For this review, take the finished solid that the model builds, in its own axes (mm). A direction names the side the tool comes from. Give positions to 0.01 mm unless a question says otherwise; leave off trailing zeros. Loops run counter-clockwise (first coordinate to the right, second up) from the corner with the lowest first, then second, coordinate; pieces in that order, holes last. Notation, with made-up numbers: (84.5, 72.5) - (141.5, 72.5) arc R24 ccw to (141.5, 98.5) - close; hole circle Ø1 at (26.25, -16.75). An arc over 180 degrees is marked (long way). Put each result on its own line as item: value.
from build123d import *

# Parameters (mm, degrees)
ESQUISSE1_R             = 1.75
ESQUISSE1_R_2           = 3.5
BOSS_EXTRU_1_DEPTH      = 5
ENL_V_MAT_EXTRU_2_REACH = 41.592
BOSS_EXTRU_2_DEPTH      = 30
ESQUISSE5_W             = 30
ESQUISSE5_H             = 5
BOSS_EXTRU_3_DEPTH      = 20
BOSS_EXTRU_4_DEPTH      = 2
BOSS_EXTRU_5_DEPTH      = 2
ENL_V_MAT_EXTRU_3_REACH = 42.516
ESQUISSE12_R            = 1.75
BOSS_EXTRU_6_DEPTH      = 4
BOSS_EXTRU_6_DEPTH_BACK = 4


with BuildPart() as part:
    # Esquisse1 → Boss.-Extru.1 (new body)
    with BuildSketch(Plane.XY):
        with BuildLine():
            Line((-15.959557324, 10.348837209), (-15.959557324, -9.651162791))
            Line((-15.959557324, -9.651162791), (14.040442676, -9.651162791))
            Line((14.040442676, -9.651162791), (14.040442676, 10.348837209))
            ThreePointArc((14.040442676, 10.348837209), (-0.959557324, 25.348837209), (-15.959557324, 10.348837209))
        make_face()
        with Locations((-8.959557324, 10.348837209)):
            Circle(ESQUISSE1_R, mode=Mode.SUBTRACT)
        with Locations((7.040442676, 10.348837209)):
            Circle(ESQUISSE1_R, mode=Mode.SUBTRACT)
        with Locations((-0.959557324, 10.348837209)):
            Circle(ESQUISSE1_R_2, mode=Mode.SUBTRACT)
    extrude(amount=BOSS_EXTRU_1_DEPTH)

    # Esquisse2 → Enlèv. mat.-Extru.2 (cut, up to next)
    with BuildSketch(Plane.ZY.offset(15.959557324), mode=Mode.PRIVATE) as enl_v_mat_extru_2_sk1:
        Polygon((0, -9.651162791), (0, -6.1501251), (1.274273509, -9.651162791), align=None)
    enl_v_mat_extru_2_tool1 = extrude(enl_v_mat_extru_2_sk1.sketch, amount=-ENL_V_MAT_EXTRU_2_REACH, mode=Mode.PRIVATE) & part.part
    add(enl_v_mat_extru_2_tool1.solids().sort_by_distance((-15.959557, -8.48415, 0.424758))[0], mode=Mode.SUBTRACT)

    # Esquisse4 → Boss.-Extru.2 (add)
    with BuildSketch(Plane.ZY.offset(15.959557324)):
        Polygon((5, -9.651162791), (1.710100717, -10.848588204), (1.274273509, -9.651162791), align=None)
    extrude(amount=-BOSS_EXTRU_2_DEPTH)

    # Esquisse5 → Boss.-Extru.3 (add)
    with BuildSketch(Plane(origin=(0, -0.719427971, -1.976612106), x_dir=(-1, 0, 0), z_dir=(0, -0.34202014332566333, -0.9396926207859103))):
        with Locations((0.959557324, -8.279227173)):
            Rectangle(ESQUISSE5_W, ESQUISSE5_H)
    extrude(amount=BOSS_EXTRU_3_DEPTH)

    # Esquisse6 → Boss.-Extru.4 (add)
    with BuildSketch(Plane.ZY.offset(15.959557324)):
        with BuildLine():
            Line((0, 10.348837209), (0, -6.1501251))
            Line((0, -6.1501251), (-18.793852416, -12.990527966))
            add(Edge.make_bspline(
                [(0, 10.348837209), (0, 0.360316824), (-21.221447274, -6.32076591), (-18.793852416, -12.990527966)],
                knots=[0, 0, 0, 0, 1, 1, 1, 1], degree=3))
        make_face()
    extrude(amount=-BOSS_EXTRU_4_DEPTH)

    # Esquisse11 → Boss.-Extru.5 (add)
    with BuildSketch(Plane.ZY.offset(-14.040442676)):
        with BuildLine():
            Line((0, 10.348837209), (0, -6.1501251))
            Line((0, -6.1501251), (-18.793852416, -12.990527966))
            add(Edge.make_bspline(
                [(0, 10.348837209), (0, 0.360316824), (-21.221447274, -6.32076591), (-18.793852416, -12.990527966)],
                knots=[0, 0, 0, 0, 1, 1, 1, 1], degree=3))
        make_face()
    extrude(amount=BOSS_EXTRU_5_DEPTH)

    # Esquisse12 → Enlèv. mat.-Extru.3 (cut, up to next)
    with BuildSketch(Plane(origin=(0, -5.430697128, 1.976612106), x_dir=(1, 0, 0), z_dir=(0, 0.9396926207859103, -0.34202014332566333)), mode=Mode.PRIVATE) as enl_v_mat_extru_3_sk1:
        with Locations(Location((-9.959557324, 18.103466668, 0), (0, 0, 270))):
            Circle(ESQUISSE12_R)
    enl_v_mat_extru_3_tool1 = extrude(enl_v_mat_extru_3_sk1.sketch, amount=-ENL_V_MAT_EXTRU_3_REACH, mode=Mode.PRIVATE) & part.part
    # Esquisse12 → Enlèv. mat.-Extru.3 (cut, up to next)
    with BuildSketch(Plane(origin=(0, -5.430697128, 1.976612106), x_dir=(1, 0, 0), z_dir=(0, 0.9396926207859103, -0.34202014332566333)), mode=Mode.PRIVATE) as enl_v_mat_extru_3_sk2:
        with Locations(Location((8.040442676, 18.103466668, 0), (0, 0, 270))):
            Circle(ESQUISSE12_R)
    enl_v_mat_extru_3_tool2 = extrude(enl_v_mat_extru_3_sk2.sketch, amount=-ENL_V_MAT_EXTRU_3_REACH, mode=Mode.PRIVATE) & part.part
    # Esquisse12 → Enlèv. mat.-Extru.3 (cut, up to next)
    with BuildSketch(Plane(origin=(0, -5.430697128, 1.976612106), x_dir=(1, 0, 0), z_dir=(0, 0.9396926207859103, -0.34202014332566333)), mode=Mode.PRIVATE) as enl_v_mat_extru_3_sk3:
        with Locations(Location((8.040442676, 6.103466668, 0), (0, 0, 270))):
            Circle(ESQUISSE12_R)
    enl_v_mat_extru_3_tool3 = extrude(enl_v_mat_extru_3_sk3.sketch, amount=-ENL_V_MAT_EXTRU_3_REACH, mode=Mode.PRIVATE) & part.part
    # Esquisse12 → Enlèv. mat.-Extru.3 (cut, up to next)
    with BuildSketch(Plane(origin=(0, -5.430697128, 1.976612106), x_dir=(1, 0, 0), z_dir=(0, 0.9396926207859103, -0.34202014332566333)), mode=Mode.PRIVATE) as enl_v_mat_extru_3_sk4:
        with Locations(Location((-9.959557324, 6.103466668, 0), (0, 0, 270))):
            Circle(ESQUISSE12_R)
    enl_v_mat_extru_3_tool4 = extrude(enl_v_mat_extru_3_sk4.sketch, amount=-ENL_V_MAT_EXTRU_3_REACH, mode=Mode.PRIVATE) & part.part
    add(enl_v_mat_extru_3_tool1.solids().sort_by_distance((-9.959557, -11.622447, -15.035082))[0], mode=Mode.SUBTRACT)
    add(enl_v_mat_extru_3_tool2.solids().sort_by_distance((8.040443, -11.622447, -15.035082))[0], mode=Mode.SUBTRACT)
    add(enl_v_mat_extru_3_tool3.solids().sort_by_distance((8.040443, -7.518206, -3.75877))[0], mode=Mode.SUBTRACT)
    add(enl_v_mat_extru_3_tool4.solids().sort_by_distance((-9.959557, -7.518206, -3.75877))[0], mode=Mode.SUBTRACT)

    # Esquisse16 → Boss.-Extru.6 (add, two sides: drawn at the far end of the back side and taken through both)
    with BuildSketch(Plane(origin=(-0.959557324, 0, 0), x_dir=(0, 0, -1), z_dir=(1, 0, 0)).offset(-BOSS_EXTRU_6_DEPTH_BACK)):
        Polygon((18.793852416, -12.990527966), (0, -6.1501251), (0, -2.534631071), align=None)
    extrude(amount=BOSS_EXTRU_6_DEPTH + BOSS_EXTRU_6_DEPTH_BACK)


solid = part.part
1) Take a section at A-A on x = 7. State the section outline as (y, z) points.
Geometry check:
outline: (-17.69, -17.08) - (-12.99, -18.79) - (-12.1, -16.36) - (-16.8, -14.65) - close; (-15.84, -12) - (-11.14, -13.71) - (-8, -5.08) - (-12.7, -3.37) - close; (-11.74, -0.73) - (-7.04, -2.44) - (-6.15, 0) - (8.6, 0) - (8.6, 5) - (-9.65, 5) - close; (12.1, 0) - (23.06, 0) - (23.06, 5) - (12.1, 5) - close
2) For faces 1 (the face through (-4.96, -7, -6)), 2 (the face through (9.52, -13.62, -13.31)), list the 3-axis set-ups (+Z, -Z, +X, -X, +Y, -Y) from which the entire face can be reached by the end or side of a thin tool; tool diameter is ignored.
Geometry check:
face 1: -Z, +Y
face 2: none
3) Wall thickness on line 1 (X direction, y = -6, z = -7.5); line 2 (Y direction, x = -3.5, z = 3.25); line 3 (Z direction, x = 2, y = 13): over which ranges is each line inside the solid? List them lowest first.
Geometry check:
line 1: x = -15.96 to -13.96, 12.04 to 14.04
line 2: y = -10.29 to 7.94, 12.76 to 25.13
line 3: z = 0 to 5
4) Take a section at B-B on x = 0. State the section outline as (y, z) points.
Geometry check:
outline: (-17.69, -17.08) - (-12.99, -18.79) - (-2.53, 0) - (6.98, 0) - (6.98, 5) - (-9.65, 5) - close; (13.71, 0) - (25.32, 0) - (25.32, 5) - (13.71, 5) - close
5) Insertion check: pin 1 Ø5 at (x, z) = (5.5, -1) entering from -Y; pin 2 Ø10 at (y, z) = (4, -11.5) entering from +X; pin 3 Ø8 at (x, y) = (-0.96, 10.35) entering from +Z; pin 4 Ø15 at (x, y) = (-1, 8) entering from -Z. Each pin has a flat end and moves straight along its axis. Give the tip position at first contact, or say it passes through.
Geometry check:
pin 1: stops at y = -12.74
pin 2: passes through
pin 3: stops at z = 5
pin 4: stops at z = 0
6) Draft analysis for pull direction Y (two halves, no side actions). For faces 3 (the face through (-4.456, 10.503, 2.465)), 4 (the face through (12.04, -5, -7)), 5 (the face through (-0.75, -15.31, -17.95)), state which applies: pulls with the +Y half, pulls with the -Y half, needs draft (parallel to the pull), parting line crosses it, or undercut.
Geometry check:
face 3: undercut
face 4: needs draft
face 5: pulls with the -Y half
7) Take a section at C-C on z = -14. State how many separate pieces and enclosed holes the cut face has, and give its area (3 significant figures).
Geometry check:
separate pieces: 3
enclosed holes: 0
area: 155 mm²
